For this review, take the finished solid that the model builds, in its own axes (mm). A direction names the side the tool comes from. Round coordinates to 2 decimals unless told otherwise and drop trailing zeros. Order: outer loops, then holes, each group sorted by start corner. A loop starts at its lowest first (then second) coordinate and runs counter-clockwise, first axis right, second up. Notation, with made-up numbers: M 70.25,-4.75 L 92.25,-4.75 A13 cw 92.25,18.25 Z; hole C 4,58.5 d2. An arc over 180 degrees is marked long. Put each result on its own line as item: value.
from build123d import *

# Parameters (mm, degrees)
BOSS_EXTRUDE1_DEPTH     = 55
CUT_EXTRUDE1_DEPTH      = 81.156097709
CUT_EXTRUDE1_DEPTH_BACK = 81.156097709
SKETCH2_W               = 70
SKETCH2_H               = 60
CUT_EXTRUDE4_DEPTH      = 125.49899598
CUT_EXTRUDE4_DEPTH_BACK = 125.49899598
SKETCH5_R               = 15
FILLET1_R               = 5
CUT_EXTRUDE5_DEPTH      = 87.746757864
CUT_EXTRUDE5_DEPTH_BACK = 87.746757864
SKETCH6_R               = 15


with BuildPart() as part:
    # Sketch1 → Boss-Extrude1 (new, symmetric)
    with BuildSketch(Plane(origin=(0, 0, 0), x_dir=(0, 0, -1), z_dir=(1, 0, 0))):
        with BuildLine():
            Line((0, 30), (50, 30))
            Line((50, 30), (50, -30))
            Line((50, -30), (0, -30))
            ThreePointArc((0, -30), (-30, 0), (0, 30))
        make_face()
    extrude(amount=BOSS_EXTRUDE1_DEPTH, both=True)

    # Sketch2 → Cut-Extrude1 (cut, two sides: drawn at the far end of the back side and taken through both)
    with BuildSketch(Plane(origin=(0, 0, 0), x_dir=(1, 0, 0), z_dir=(0, 1, 0)).offset(-CUT_EXTRUDE1_DEPTH_BACK)):
        Rectangle(SKETCH2_W, SKETCH2_H)
    extrude(amount=CUT_EXTRUDE1_DEPTH + CUT_EXTRUDE1_DEPTH_BACK, mode=Mode.SUBTRACT)

    # Sketch5 → Cut-Extrude4 (cut, two sides: drawn at the far end of the back side and taken through both)
    with BuildSketch(Plane.ZY.offset(55).offset(-CUT_EXTRUDE4_DEPTH_BACK)):
        Circle(SKETCH5_R)
    extrude(amount=CUT_EXTRUDE4_DEPTH + CUT_EXTRUDE4_DEPTH_BACK, mode=Mode.SUBTRACT)

    # Fillet1
    fillet1_edges = [part.edges().sort_by_distance(p)[0] for p in [
        (55, 0, -50),
        (35, 0, -30),
        (-35, 0, -30),
        (-55, 0, -50),
    ]]
    fillet(fillet1_edges, radius=FILLET1_R)

    # Sketch6 → Cut-Extrude5 (cut, two sides: drawn at the far end of the back side and taken through both)
    with BuildSketch(Plane.XY.offset(-30).offset(-CUT_EXTRUDE5_DEPTH_BACK)):
        Circle(SKETCH6_R)
    extrude(amount=CUT_EXTRUDE5_DEPTH + CUT_EXTRUDE5_DEPTH_BACK, mode=Mode.SUBTRACT)


solid = part.part
(1) Insertion check: pin 1 Ø2 at (y, z) = (12.5, 6) entering from +X; pin 2 Ø18 at (x, y) = (-4, -7.5) entering from +Z. Each pin has a flat end and moves straight along its axis. Give the tip position at first contact, or say it passes through.
A:
pin 1: passes through
pin 2: stops at z = -30
(2) Add section A-A on y = 0. Give the boundary of the cut face in (x, z), then the cut area to 3 significant figures.
A:
outline: M -55,-45 A5 ccw -50,-50 L -15,-50 L -15,-30 L -30,-30 A5 cw -35,-25 L -35,-15 L -55,-15 Z; M -55,15 L -35,15 L -35,30 L -55,30 Z; M 15,-50 L 50,-50 A5 ccw 55,-45 L 55,-15 L 35,-15 L 35,-25 A5 cw 30,-30 L 15,-30 Z; M 35,15 L 55,15 L 55,30 L 35,30 Z
area: 2,800 mm2
(3) Add section B-B on x = 0. Give the boundary of the cut face in (y, z).
A:
outline: M -30,-50 L -15,-50 L -15,-30 L -30,-30 Z; M 15,-50 L 30,-50 L 30,-30 L 15,-30 Z
(4) Draft analysis for pull direction Y (two halves, no side actions). For faces 1 (the face through (-44.86, 0.66, -14.985)), 2 (the face through (-44.86, -0.66, 29.993)), 3 (the face through (0.8, 30, -30.2)), 4 (the face through (12, 14, -50)), state which applies: released by +Y, released by -Y, zero draft, split by the parting line, or undercut.
A:
face 1: undercut
face 2: split by the parting line
face 3: released by +Y
face 4: zero draft
(5) For faces 5 (the face through (54, 0, -48)), 6 (the face through (-34, 0, -28)), list the 3-axis set-ups (+Z, -Z, +X, -X, +Y, -Y) from which the entire face can be reached by the end or side of a thin tool; tool diameter is ignored.
A:
face 5: -Z, +X, +Y, -Y
face 6: +Z, +Y, -Y
(6) Add section D-D on x = -45.5. Give the boundary of the cut face in (y, z).
A:
outline: M -30,-50 L 30,-50 L 30,0 A30 ccw -30,0 Z; hole C 0,0 d30
(7) Add section C-C on z = -20. Give the boundary of the cut face in (x, y).
A:
outline: M -55,-30 L -35,-30 L -35,30 L -55,30 Z; M 35,-30 L 55,-30 L 55,30 L 35,30 Z
(8) To check wall thickness, follow L1, parallel to X at y = 0, z = -42.5; L2, parallel to X at y = -9.5, z = -16; L3, parallel to Y at x = 0, z = -36.25. State the ranges of each line that lie inside material, in increasing order.
A:
L1: x = -55 to -15, 15 to 55
L2: x = -55 to -35, 35 to 55
L3: y = -30 to -15, 15 to 30
